Could you check a few things on this model? Use its own coordinates, in mm. Round coordinates to 2 decimals unless told otherwise and drop trailing zeros. Loops run counter-clockwise (first coordinate to the right, second up) from the corner with the lowest first, then second, coordinate; pieces in that order, holes last. Notation, with made-up numbers: (15, 33.5) - (40, 33.5) arc R3 ccw to (40, 38.5) - close; hole circle Ø1 at (39, -0.5). An arc over 180 degrees is marked (long way). Answer as CSV lines item,"result". Start each with the question number.
1) I'm going to push a flat-ended pin straight in: pin 1 Ø2 at (x, z) = (3, 303.5) entering from +Y. Where does the tip first touch, or does it pass through?
2) Please list where these lines run through material, in increasing order: line 1 along Y through (x, z) = (0, 541.5); line 2 along X through (y, z) = (0.5, 155); line 3 along Y through (x, z) = (-1.75, 498.5).
3) Suppose I cut it at A-A, the plane z = 132. Write out the boundary of the cut face in (x, y).
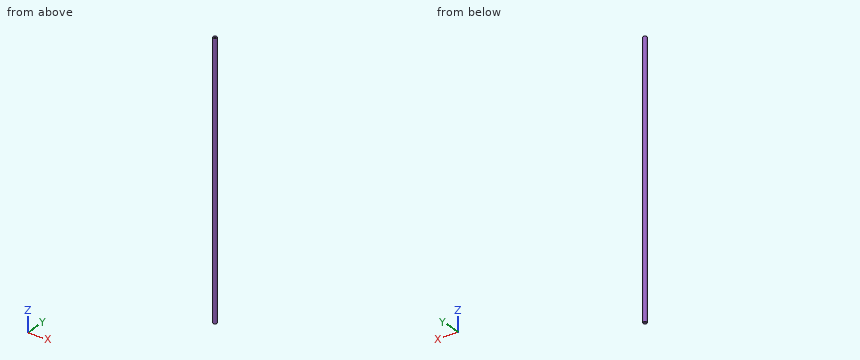
```python
from build123d import *

# Parameters (mm, degrees)
SKETCH1_R           = 4
BOSS_EXTRUDE1_DEPTH = 544
SKETCH2_R           = 1
CUT_EXTRUDE1_DEPTH  = 10
CHAMFER1_SIZE       = 0.5


with BuildPart() as part:
    # Sketch1 → Boss-Extrude1 (new body)
    with BuildSketch(Plane.XY):
        Circle(SKETCH1_R)
    extrude(amount=BOSS_EXTRUDE1_DEPTH)

    # Sketch2 → Cut-Extrude1 (cut)
    with BuildSketch(Plane.XY.offset(544)):
        Circle(SKETCH2_R)
    extrude(amount=-CUT_EXTRUDE1_DEPTH, mode=Mode.SUBTRACT)

    # Chamfer1
    chamfer1_edges = [part.edges().sort_by_distance(p)[0] for p in [
        (-4, 0, 0),
        (-4, 0, 544),
    ]]
    chamfer(chamfer1_edges, length=CHAMFER1_SIZE)


solid = part.part
```
Filled sheet:
1,pin 1,"y = 3.46"
2,line 1,"-4 to -1, 1 to 4"
2,line 2,"-3.97 to 3.97"
2,line 3,"-3.6 to 3.6"
3,outline,"circle Ø8 at (0, 0)"
